Here's how the part is built. I have some questions about the finished solid (model axes, mm). Round coordinates to 2 decimals unless told otherwise and drop trailing zeros. Loops run counter-clockwise (first coordinate to the right, second up) from the corner with the lowest first, then second, coordinate; pieces in that order, holes last. Notation, with made-up numbers: M -39,63.25 L 8,63.25 A23 cw 8,100.25 Z; hole C 86,33 d3. An arc over 180 degrees is marked long. Answer as CSV lines item,"result".
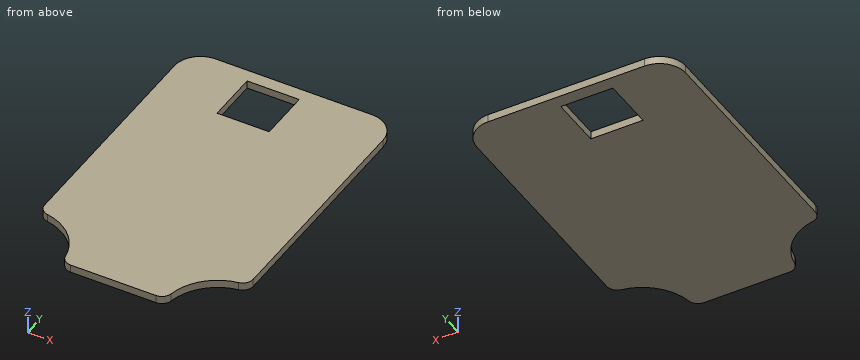
```python
from build123d import *

# Parameters (mm, degrees)
F0_W     = 25.4
F0_H     = 25.4
F1_DEPTH = 3.81
F2_R     = 5.08
F3_R     = 5.08
F4_R     = 12.7


with BuildPart() as f1:
    # F0 (on Top) → F1 (new body)
    with BuildSketch(Plane.XY):
        with BuildLine():
            Line((-12.7, 96.302761), (-57.15, 96.302761))
            Line((-57.15, 96.302761), (-57.15, 89.952761))
            Line((-57.15, 89.952761), (-57.15, 83.602761))
            Line((-57.15, 83.602761), (-57.15, 70.902761))
            Line((-57.15, 70.902761), (-57.15, -30.697239))
            ThreePointArc((-57.15, -30.697239), (-39.189488, -38.136727), (-31.75, -56.097239))
            Line((-31.75, -56.097239), (19.05, -56.097239))
            ThreePointArc((19.05, -56.097239), (26.489488, -38.136727), (44.45, -30.697239))
            Line((44.45, -30.697239), (44.45, 96.302761))
            Line((44.45, 96.302761), (0, 96.302761))
            Line((0, 96.302761), (-12.7, 96.302761))
        make_face()
        with Locations((-12.7, 77.252761)):
            Rectangle(F0_W, F0_H, mode=Mode.SUBTRACT)
    extrude(amount=F1_DEPTH)

    # F2
    f2_edges = [f1.edges().sort_by_distance(p)[0] for p in [
        (-57.15, -30.697239, 1.905),
        (-31.75, -56.097239, 1.905),
    ]]
    fillet(f2_edges, radius=F2_R)

    # F3
    f3_edges = [f1.edges().sort_by_distance(p)[0] for p in [
        (44.45, -30.697239, 1.905),
        (19.05, -56.097239, 1.905),
    ]]
    fillet(f3_edges, radius=F3_R)

    # F4
    f4_edges = [f1.edges().sort_by_distance(p)[0] for p in [
        (-57.15, 96.302761, 1.905),
        (44.45, 96.302761, 1.905),
    ]]
    fillet(f4_edges, radius=F4_R)


solid = f1.part
```
1. If I drill on line 1 (X direction, y = 86, z = 2.75); line 2 (Y direction, x = -34, z = 2.75); line 3 (Y direction, x = 21, z = 3.5), over which ranges is the centre line in solid material (lowest first)? Write a range as [from, to].
Evaluation:
line 1,"x = [-56.92, -25.4], [0, 44.22]"
line 2,"y = [-45.65, 96.3]"
line 3,"y = [-46.34, 96.3]"
2. For P1, Ø6, axis at x = 22.5, y = -35.5, coming from the -Z side, with a flat end and sliding along its axis, tell me the tip position at first contact or that it passes through.
Evaluation:
P1,"stops at z = 0"
3. I want a section at C-C, the plane x = -46.5. Please give me the cut outline in (y, z).
Evaluation:
outline,"M -33.04,0 L 96.14,0 L 96.14,3.81 L -33.04,3.81 Z"
4. I want a section at A-A, the plane x = -4. Please give me the cut outline in (y, z).
Evaluation:
outline,"M -56.1,0 L 64.55,0 L 64.55,3.81 L -56.1,3.81 Z; M 89.95,0 L 96.3,0 L 96.3,3.81 L 89.95,3.81 Z"
5. I want a section at B-B, the plane z = 3.1. Please give me the cut outline in (x, y).
Evaluation:
outline,"M -57.15,-26.04 A5.08 ccw -52.92,-31.05 A25.4 cw -32.11,-51.86 A5.08 ccw -27.1,-56.1 L 14.4,-56.1 A5.08 ccw 19.41,-51.86 A25.4 cw 40.22,-31.05 A5.08 ccw 44.45,-26.04 L 44.45,83.6 A12.7 ccw 31.75,96.3 L -44.45,96.3 A12.7 ccw -57.15,83.6 Z; hole M -25.4,64.55 L 0,64.55 L 0,89.95 L -25.4,89.95 Z"
